Design review of the part built by this model. Coordinates are the model's own, in mm. Face numbers are marked on the shaded views. A direction names the side the tool comes from. Coordinates: 2 decimals unless noted, no trailing zeros. Loops run counter-clockwise (first coordinate to the right, second up) from the corner with the lowest first, then second, coordinate; pieces in that order, holes last. Notation, with made-up numbers: (-1.75, -13.75) -> (18.25, -13.75) arc R9 cw to (18.25, -9.75) -> close; hole circle Ø8 at (5, 76.5). An arc over 180 degrees is marked (long way). Use one line per item in the form item = value. Start each with the question number.
1. The part is to be moulded in two halves that separate along Y. For the marked faces 1, 2 and 3, say which applies: released by +Y, released by -Y, zero draft, split by the parting line, or undercut.
2. Consider section B-B (y = -0.75). State the section outline as (x, z) points.
3. Machinability: for the marked faces 4 and 5, which of the approach directions +Z, -Z, +X, -X, +Y, -Y give a long, thin tool a straight path to every point of the face, cutting with its end or side? Answer none if there is none.
4. Consider section A-A (x = 14). State the section outline as (y, z) points.
5. Wall thickness on line 1 (X direction, y = 0.75, z = 1.5); line 2 (Y direction, x = 27, z = -5); line 3 (Y direction, x = 20, z = -15): over which ranges is each line inside the solid? List them lowest first. Write a range as from..to.
6. For pin 1 (2 mm diameter, centred on x = 19.5, y = -5.5, fed in from -Z); pin 2 (3 mm diameter, centred on x = -19, y = 1, fed in from -Z), all flat-tipped, find the tip position at first contact; note any pin that passes through.
from build123d import *

# Parameters (mm, degrees)
BOSS_EXTRUDE1_DEPTH      = 7.5
BOSS_EXTRUDE1_DEPTH_BACK = 7.5
SKETCH1_W                = 75
SKETCH1_H                = 40
CUT_EXTRUDE1_DEPTH       = 5.2
CUT_EXTRUDE1_DEPTH_BACK  = 20
CHAMFER1_SIZE            = 2
SKETCH3_R                = 2
CUT_EXTRUDE2_DEPTH       = 9
CUT_EXTRUDE3_DEPTH       = 4.7
FILLET1_R                = 2


with BuildPart() as part:
    # Sketch1 → Boss-Extrude1 (new, two sides: drawn at the far end of the back side and taken through both)
    with BuildSketch(Plane(origin=(0, 0, 0), x_dir=(1, 0, 0), z_dir=(0, 1, 0)).offset(-BOSS_EXTRUDE1_DEPTH_BACK)):
        Rectangle(SKETCH1_W, SKETCH1_H)
    extrude(amount=BOSS_EXTRUDE1_DEPTH + BOSS_EXTRUDE1_DEPTH_BACK)

    # Sketch2 → Cut-Extrude1 (cut, two sides: drawn at the far end of the back side and taken through both)
    with BuildSketch(Plane.XY.offset(-CUT_EXTRUDE1_DEPTH_BACK)):
        with BuildLine():
            Line((6.87897019, 18.765118011), (-6.87897019, 18.765118011))
            add(Edge.make_bspline(
                [(-6.87897019, 18.765118011), (-9.129399026, 18.205247728), (-11.266061827, 17.3684432), (-15.104945109, 15.221192023), (-16.806572871, 13.91106443), (-19.608554315, 10.943595702), (-20.708442739, 9.286661987), (-22.197433977, 5.786794286), (-22.586183082, 3.944422776), (-22.599635329, 2.1)],
                knots=[0, 0, 0, 0, 0.25, 0.25, 0.5, 0.5, 0.75, 0.75, 1, 1, 1, 1], degree=3))
            Line((-22.599635329, 2.1), (-27.6, 2.1))
            Line((-27.6, 2.1), (-27.6, -2.1))
            Line((-27.6, -2.1), (-21.5, -2.1))
            Line((-21.5, -2.1), (-18.5, -2.1))
            Line((-18.5, -2.1), (-12.4, -2.1))
            Line((-12.4, -2.1), (-12.4, 2.1))
            Line((-12.4, 2.1), (-17.399433648, 2.1))
            add(Edge.make_bspline(
                [(-17.399433648, 2.1), (-17.381202069, 3.709535833), (-16.917608437, 5.316341272), (-15.60243407, 7.545915267), (-15.061738812, 8.259029365), (-13.79568918, 9.597737471), (-13.070365792, 10.223287356), (-10.658457879, 11.932196217), (-8.73364722, 12.845140962), (-4.538397278, 14.079281106), (-2.269643886, 14.4), (2.269643886, 14.4), (4.538397278, 14.079281106), (8.73364722, 12.845140962), (10.658457879, 11.932196217), (13.070365792, 10.223287356), (13.79568918, 9.597737471), (15.061738812, 8.259029365), (15.60243407, 7.545915267), (16.917608437, 5.316341272), (17.381202069, 3.709535833), (17.399433648, 2.1)],
                knots=[0, 0, 0, 0, 0.125, 0.125, 0.1875, 0.1875, 0.25, 0.25, 0.375, 0.375, 0.5, 0.5, 0.625, 0.625, 0.75, 0.75, 0.8125, 0.8125, 0.875, 0.875, 1, 1, 1, 1], degree=3))
            Line((17.399433648, 2.1), (12.4, 2.1))
            Line((12.4, 2.1), (12.4, -2.1))
            Line((12.4, -2.1), (18.5, -2.1))
            Line((18.5, -2.1), (21.5, -2.1))
            Line((21.5, -2.1), (27.6, -2.1))
            Line((27.6, -2.1), (27.6, 2.1))
            Line((27.6, 2.1), (22.599635329, 2.1))
            add(Edge.make_bspline(
                [(22.599635329, 2.1), (22.586183082, 3.944422776), (22.197433977, 5.786794286), (20.708442739, 9.286661987), (19.608554315, 10.943595702), (16.806572871, 13.91106443), (15.104945109, 15.221192023), (11.266061827, 17.3684432), (9.129399026, 18.205247728), (6.87897019, 18.765118011)],
                knots=[0, 0, 0, 0, 0.25, 0.25, 0.5, 0.5, 0.75, 0.75, 1, 1, 1, 1], degree=3))
        make_face()
    extrude(amount=CUT_EXTRUDE1_DEPTH + CUT_EXTRUDE1_DEPTH_BACK, mode=Mode.SUBTRACT)

    # Chamfer1
    chamfer1_edges = [part.edges().sort_by_distance(p)[0] for p in [
        (-16.904241207, 4.934871199, 5.2),
        (-22.30006804, 4.855503871, 5.2),
        (22.30006804, 4.855503871, 5.2),
        (16.904241207, 4.934871199, 5.2),
    ]]
    chamfer(chamfer1_edges, length=CHAMFER1_SIZE)

    # Sketch3 → Cut-Extrude2 (cut)
    with BuildSketch(Plane(origin=(0, 0, -20), x_dir=(-1, 0, 0), z_dir=(0, 0, -1))):
        with Locations((-20, -4.8)):
            Circle(SKETCH3_R)
        with Locations(Location((20, -4.8, 0), (0, 0, 180))):
            Circle(SKETCH3_R)
    extrude(amount=-CUT_EXTRUDE2_DEPTH, mode=Mode.SUBTRACT)

    # Sketch4 → Cut-Extrude3 (cut)
    with BuildSketch(Plane(origin=(0, -2.1, 0), x_dir=(1, 0, 0), z_dir=(0, 1, 0))):
        with BuildLine():
            Line((-22, 7.5), (-22, 10))
            Line((-22, 10), (-18, 10))
            Line((-18, 10), (-18, 7.5))
            ThreePointArc((-18, 7.5), (-20, 5.5), (-22, 7.5))
        make_face()
        with BuildLine():
            Line((18, 10), (18, 7.5))
            ThreePointArc((18, 7.5), (20, 5.5), (22, 7.5))
            Line((22, 7.5), (22, 10))
            Line((22, 10), (18, 10))
        make_face()
    extrude(amount=-CUT_EXTRUDE3_DEPTH, mode=Mode.SUBTRACT)

    # Fillet1
    fillet1_edges = [part.edges().sort_by_distance(p)[0] for p in [
        (-22, -6.8, -8.75),
        (-18, -6.8, -8.75),
        (-20, -6.8, -5.5),
        (18, -6.8, -8.75),
        (22, -6.8, -8.75),
        (20, -6.8, -5.5),
    ]]
    fillet(fillet1_edges, radius=FILLET1_R - 0.0001)  # a hair under: the kernel refuses the full size


solid = part.part
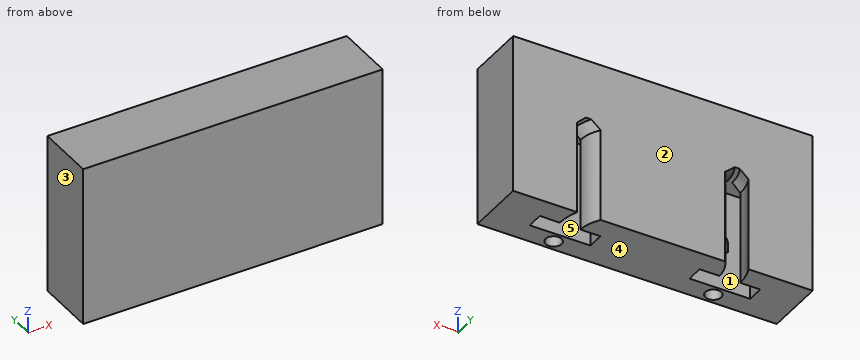
Geometry check:
q1.face_1 = undercut
q1.face_2 = released by +Y
q1.face_3 = zero draft
q2.outline = (-37.5, -20) -> (-27.6, -20) -> (-27.6, 5.2) -> (-12.4, 5.2) -> (-12.4, -20) -> (12.4, -20) -> (12.4, 5.2) -> (27.6, 5.2) -> (27.6, -20) -> (37.5, -20) -> (37.5, 20) -> (-37.5, 20) -> close
q3.face_4 = -Z, +X, -X, +Y, -Y
q3.face_5 = -Z
q4.outline = (-7.5, -20) -> (-2.1, -20) -> (-2.1, 5.2) -> (2.1, 5.2) -> (2.1, -20) -> (7.5, -20) -> (7.5, 20) -> (-7.5, 20) -> close
q5.line_1 = -37.5..-27.6, -12.4..12.4, 27.6..37.5
q5.line_2 = -7.5..-2.1, 2.1..7.5
q5.line_3 = -7.5..-6.8, -2.8..-2.1
q6.pin_1 = -11
q6.pin_2 = 3.78
